Here's how the part is built. I have some questions about the finished solid (model axes, mm). A direction names the side the tool comes from. Round coordinates to 2 decimals unless told otherwise and drop trailing zeros. Order: outer loops, then holes, each group sorted by start corner. A loop starts at its lowest first (then second) coordinate and runs counter-clockwise, first axis right, second up. Notation, with made-up numbers: (-31.5, 37) - (-9.5, 37) arc R27 ccw to (-9.5, 57) - close; hole circle Ø5 at (37.25, 46.5). An arc over 180 degrees is marked (long way). Answer as a JSON object with one key per item and string values.
```python
from build123d import *

# Parameters (mm, degrees)
ESQUISSE2_W                  = 10
ESQUISSE2_H                  = 73.61
BOSS_EXTRU_1_DEPTH           = 5
ENL_V_MAT_EXTRU_1_DEPTH      = 75.454228221
D_GAGEMENT_M31_D             = 3.4
R_P_TITION_CIRCULAIRE1_COUNT = 3
ESQUISSE8_R                  = 57.5
BOSS_EXTRU_2_DEPTH           = 10
ESQUISSE9_R                  = 47.5
ENL_V_MAT_EXTRU_3_DEPTH      = 100.437219687


with BuildPart() as part:
    # Esquisse2 → Boss.-Extru.1 (new, symmetric)
    with BuildSketch(Plane.XY):
        with Locations((0, 36.805)):
            Rectangle(ESQUISSE2_W, ESQUISSE2_H)
    boss_extru_1 = extrude(amount=BOSS_EXTRU_1_DEPTH, both=True)

    # Esquisse3 → Enlèv. mat.-Extru.1 (cut, through all)
    with BuildSketch(Plane(origin=(5, 0, 0), x_dir=(0, 0, -1), z_dir=(1, 0, 0))):
        with BuildLine():
            Line((-25.399222728, 69.089156782), (-25.399222728, 83.587655611))
            Line((-25.399222728, 83.587655611), (25.399222728, 83.587655611))
            Line((25.399222728, 83.587655611), (25.399222728, 69.089156782))
            ThreePointArc((25.399222728, 69.089156782), (0, 73.61), (-25.399222728, 69.089156782))
        make_face()
    enl_v_mat_extru_1 = extrude(amount=-ENL_V_MAT_EXTRU_1_DEPTH, mode=Mode.SUBTRACT)

    # Dégagement M31 (through all)
    with Locations(Plane(origin=(0, 0, -5), x_dir=(-1, 0, 0), z_dir=(0, 0, -1))):
        with Locations((0, 67.5)):
            d_gagement_m31 = Hole(D_GAGEMENT_M31_D / 2)

    # Répétition circulaire1: Boss.-Extru.1, Enlèv. mat.-Extru.1, Dégagement M31 ×3 about axis
    r_p_tition_circulaire1_axis = Axis((0, 0, 0), (1, 0, 0))
    add([boss_extru_1.rotate(r_p_tition_circulaire1_axis, i * 360 / R_P_TITION_CIRCULAIRE1_COUNT) for i in range(1, R_P_TITION_CIRCULAIRE1_COUNT)])
    add([enl_v_mat_extru_1.rotate(r_p_tition_circulaire1_axis, i * 360 / R_P_TITION_CIRCULAIRE1_COUNT) for i in range(1, R_P_TITION_CIRCULAIRE1_COUNT)], mode=Mode.SUBTRACT)
    add([d_gagement_m31.rotate(r_p_tition_circulaire1_axis, i * 360 / R_P_TITION_CIRCULAIRE1_COUNT) for i in range(1, R_P_TITION_CIRCULAIRE1_COUNT)], mode=Mode.SUBTRACT)

    # Esquisse8 → Boss.-Extru.2 (add)
    with BuildSketch(Plane(origin=(5, 0, 0), x_dir=(0, 0, -1), z_dir=(1, 0, 0))):
        Circle(ESQUISSE8_R)
    extrude(amount=-BOSS_EXTRU_2_DEPTH)

    # Esquisse9 → Enlèv. mat.-Extru.3 (cut, through all)
    with BuildSketch(Plane(origin=(5, 0, 0), x_dir=(0, 0, -1), z_dir=(1, 0, 0))):
        Circle(ESQUISSE9_R)
    extrude(amount=-ENL_V_MAT_EXTRU_3_DEPTH, mode=Mode.SUBTRACT)


solid = part.part
```
1. Imagine slicing it at D-D (y = 67.5). List the corners of the cut face in (x, z) for me.
Responses:
{"outline": "(-5, -5) - (-1.7, -5) - (-1.7, 5) - (-5, 5) - close; (1.7, -5) - (5, -5) - (5, 5) - (1.7, 5) - close"}
2. Imagine slicing it at A-A (z = 0). List the corners of the cut face in (x, y) for me.
Responses:
{"outline": "(-5, -57.5) - (5, -57.5) - (5, -47.5) - (-5, -47.5) - close; (-5, 47.5) - (5, 47.5) - (5, 73.61) - (-5, 73.61) - close; hole circle Ø3.4 at (0, 67.5)"}
3. Imagine slicing it at C-C (x = 0). List the corners of the cut face in (y, z) for me, plus the area to 3 significant figures.
Responses:
{"outline": "(-41.05, -61.1) arc R73.61 ccw to (-32.39, -66.1) - (-30.27, -62.43) - (-38.93, -57.43) - close; (-41.05, 61.1) - (-38.93, 57.43) - (-30.27, 62.43) - (-32.39, 66.1) arc R73.61 ccw to start; (-37.23, -54.48) - (-28.57, -59.48) - (-24.31, -52.11) arc R57.5 ccw to (57.28, -5) - (65.8, -5) - (65.8, 5) - (57.28, 5) arc R57.5 ccw to (-24.31, 52.11) - (-28.57, 59.48) - (-37.23, 54.48) - (-32.97, 47.11) arc R57.5 ccw to (-32.97, -47.11) - close; (69.2, -5) - (73.44, -5) arc R73.61 ccw to (73.44, 5) - (69.2, 5) - close; hole circle Ø95 at (0, 0)", "area": "3,680 mm2"}
4. Imagine slicing it at B-B (y = 0). List the corners of the cut face in (x, z) for me.
Responses:
{"outline": "(-5, -57.5) - (5, -57.5) - (5, -47.5) - (-5, -47.5) - close; (-5, 47.5) - (5, 47.5) - (5, 57.5) - (-5, 57.5) - close"}
5. Thinking about a two-plate mould opening in Y: for faces 1 (the face through (-0.221, -34.532, -59.951)), 2 (the face through (0, 65, 5)), 3 (the face through (0.07, 73.61, -0.07)), which applies, pulls with the +Y half, pulls with the -Y half, needs draft (parallel to the pull), parting line crosses it, or undercut?
Responses:
{"face 1": "undercut", "face 2": "needs draft", "face 3": "pulls with the +Y half"}
6. If I drill on L1, parallel to Y at x = 0, z = 0.25; L2, parallel to X at y = 67.5, z = -1.5; L3, parallel to Y at x = 0, z = -2.5, over which ranges is the centre line in solid material (lowest first)? Write a range as [from, to].
Responses:
{"L1": "[-57.5, -47.5], [47.5, 65.8], [69.2, 73.61]", "L2": "[-5, -1.7], [1.7, 5]", "L3": "[-57.45, -47.43], [47.43, 65.8], [69.2, 73.57]"}
7. For faces 4 (the face through (0, 65, -5)), 5 (the face through (-0.07, -28.407, 59.202)), 6 (the face through (-0.07, -37.067, 54.202)), which set-ups out of +Z, -Z, +X, -X, +Y, -Y let a thin tool reach every point of the face, with its end or its side?
Responses:
{"face 4": "-Z, +X, -X, +Y", "face 5": "+Z, +X, -X", "face 6": "+X, -X, -Y"}
8. For P1, Ø1, axis at x = -0.5, y = -1.5, coming from the -Z side; P2, Ø1, axis at x = 0, z = 29.5, coming from the -Y side; P3, Ø1.5, axis at x = 2, y = 45, coming from the +Z side, each with a flat end and sliding along its axis, tell me the tip position at first contact or that it passes through.
Responses:
{"P1": "z = -57.49", "P2": "y = -49.65", "P3": "z = 36.72"}
